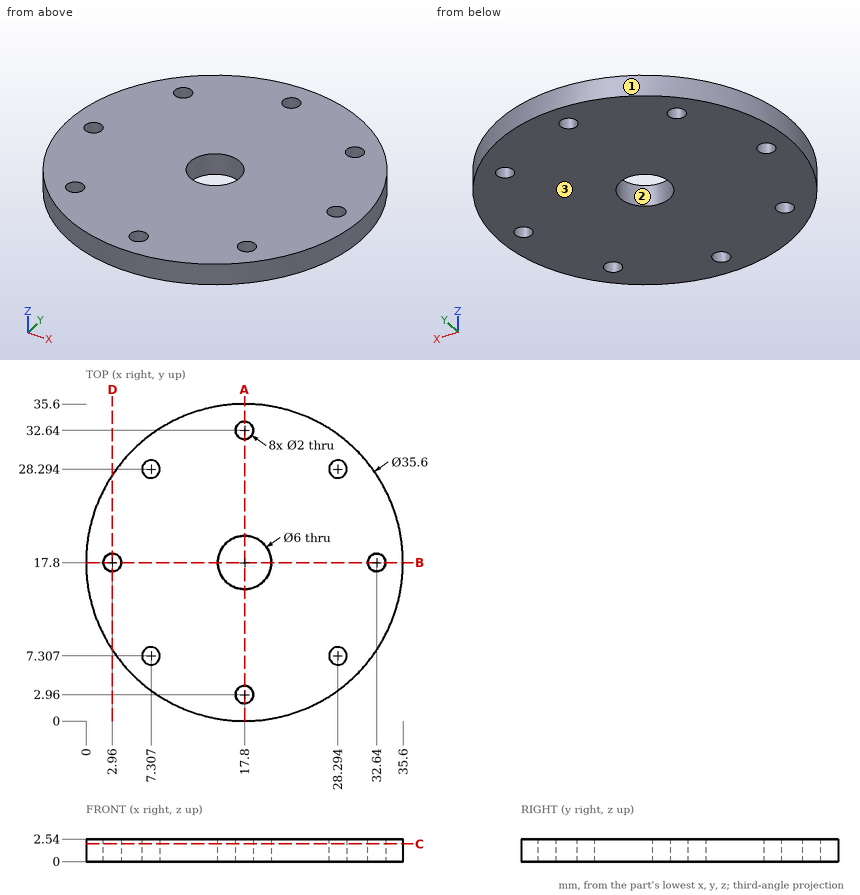
Design review of the part shown in the three views and the two pictorial views. Dimensions are in mm from the part's minimum x, y and z. Coordinates: 2 decimals unless noted, no trailing zeros. Order: outer loops, then holes, each group sorted by start corner. A loop starts at its lowest first (then second) coordinate and runs counter-clockwise, first axis right, second up. Notation, with made-up numbers: (-10.5, 81.25) - (15.5, 81.25) arc R19 ccw to (15.5, 114.25) - close; hole circle Ø4 at (51, 81.5). An arc over 180 degrees is marked (long way). Answer as CSV lines item,"result". Start each with the question number.
1) Insertion check: P1, Ø1.8, axis at x = 28.29, y = 7.31, coming from the +Z side; P2, Ø1, axis at y = 29, z = 2, coming from the +X side (1 decimal). Each pin has a flat end and moves straight along its axis. Give the tip position at first contact, or say it passes through.
2) Add section C-C (z = 2). Count the separate pieces of the cut face and the enclosed holes in it, then the cut area to 3 significant figures.
3) Add section D-D (x = 2.96). State the section outline as (y, z) points.
4) To check wall thickness, follow line 1 along Y through (x, z) = (17.8, 1.75); line 2 along X through (y, z) = (8, 0.5) (1 decimal); line 3 along Y through (x, z) = (20.5, 0.35) (1 decimal). State the ranges of each line that lie inside material, in increasing order. Write a range as [from, to].
5) Draft analysis for pull direction X (two halves, no side actions). For the marked faces 1, 2 and 3, state which applies: +X half, -X half, draft (parallel to the pull), parting line (faces both ways), or undercut.
6) Add section A-A (x = 17.8). State the section outline as (y, z) points.
Result:
1,P1,"through"
1,P2,"x = 32"
2,separate pieces,"1"
2,enclosed holes,"9"
2,area,"942 mm^2"
3,outline,"(7.97, 0) - (16.8, 0) - (16.8, 2.54) - (7.97, 2.54) - close; (18.8, 0) - (27.63, 0) - (27.63, 2.54) - (18.8, 2.54) - close"
4,line 1,"[0, 1.96], [3.96, 14.8], [20.8, 31.64], [33.64, 35.6]"
4,line 2,"[2.9, 6.6], [8, 27.6], [29, 32.7]"
4,line 3,"[0.2, 16.5], [19.1, 35.4]"
5,face 1,"parting line"
5,face 2,"undercut"
5,face 3,"draft"
6,outline,"(0, 0) - (1.96, 0) - (1.96, 2.54) - (0, 2.54) - close; (3.96, 0) - (14.8, 0) - (14.8, 2.54) - (3.96, 2.54) - close; (20.8, 0) - (31.64, 0) - (31.64, 2.54) - (20.8, 2.54) - close; (33.64, 0) - (35.6, 0) - (35.6, 2.54) - (33.64, 2.54) - close"
